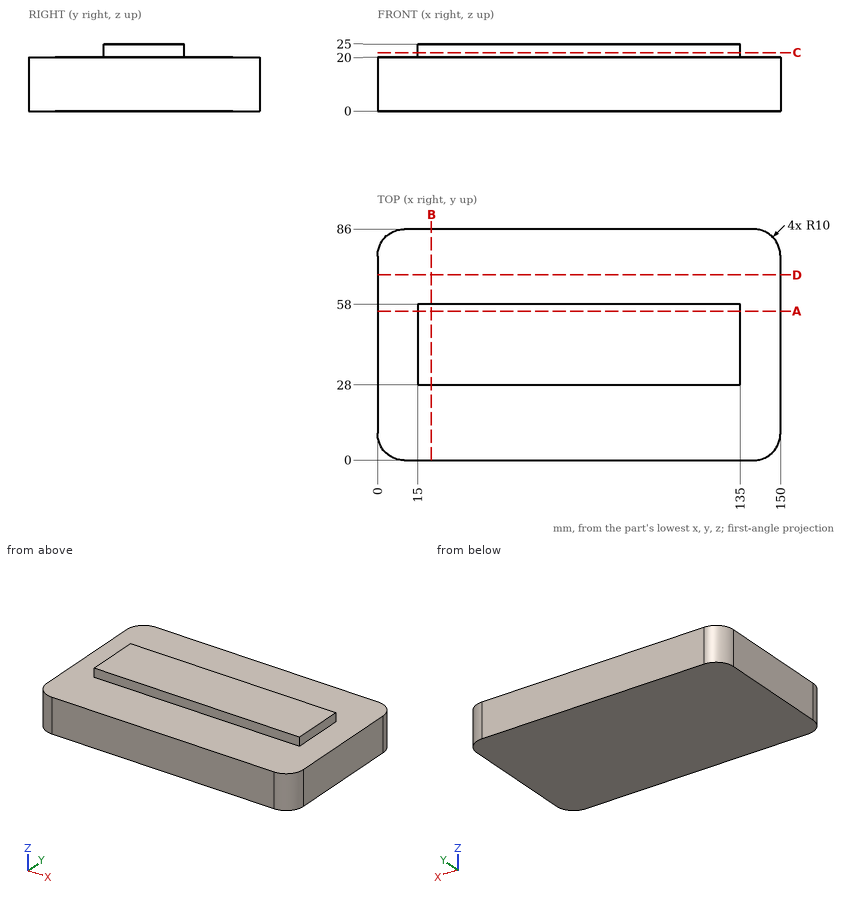
Print and shaded views of the part. All mm, measured from the part's lowest x, y and z. Give positions to 0.01 mm unless a question says otherwise; leave off trailing zeros. Write each loop counter-clockwise with the first axis right and the second up, starting at its lowest first coordinate (ties: lowest second). Pieces come first, ordered by that corner, then holes. Notation, with made-up numbers: (39, 82.25) -> (46, 82.25) arc R5 cw to (46, 90.25) -> close; hole circle Ø1 at (88, -9.5). An arc over 180 degrees is marked (long way). Write each question's results on one line, items separated by ' | '.
1. Drop flat-ended pins along their axis: P1, Ø5.5, axis at x = 92, z = 23, coming from the +Y side; P2, Ø4, axis at y = 38, z = 23.5, coming from the +X side; P3, Ø5.5, axis at x = 58.5, z = 23.5, coming from the -Y side; P4, Ø4, axis at y = 74.5, z = 22.5, coming from the +X side. Give the stop position or say it passes through.
Geometry check:
P1: y = 58 | P2: x = 135 | P3: y = 28 | P4: through
2. Wall check: probe 1 along Z at (x, y) = (62, 4.5); probe 2 along Y at (x, z) = (119, 22); probe 3 along X at (y, z) = (8, 4.5). Give the ranges that are in metal, low to high. Write a range as [from, to].
Geometry check:
probe 1: [0, 20] | probe 2: [28, 58] | probe 3: [0.2, 149.8]
3. Cut at C-C, the plane z = 21.75. Write the cut outline in (x, y).
Geometry check:
outline: (15, 28) -> (135, 28) -> (135, 58) -> (15, 58) -> close
4. Cut at B-B, the plane x = 20. Write the cut outline in (y, z).
Geometry check:
outline: (0, 0) -> (86, 0) -> (86, 20) -> (58, 20) -> (58, 25) -> (28, 25) -> (28, 20) -> (0, 20) -> close
5. Cut at A-A, the plane y = 55.5. Write the cut outline in (x, z).
Geometry check:
outline: (0, 0) -> (150, 0) -> (150, 20) -> (135, 20) -> (135, 25) -> (15, 25) -> (15, 20) -> (0, 20) -> close
6. Cut at D-D, the plane y = 69. Write the cut outline in (x, z), then the cut area to 3 significant figures.
Geometry check:
outline: (0, 0) -> (150, 0) -> (150, 20) -> (0, 20) -> close | area: 3,000 mm²
